Source: CAD feature listing. Evaluate the final solid. Frame: model axes, mm. A direction names the side the tool comes from. Give positions to 0.01 mm unless a question says otherwise; leave off trailing zeros. Order: outer loops, then holes, each group sorted by start corner. A loop starts at its lowest first (then second) coordinate and runs counter-clockwise, first axis right, second up. Notation, with made-up numbers: (48, 74) - (72, 74) arc R27 ccw to (72, 104) - close; hole circle Ø5 at (85, -8.75). An arc over 180 degrees is marked (long way). One line per item, written item: value. Start each with the question number.
Autodesk Inventor part; units mm, degrees
ref_plane "YZ Plane" through (0, 0, 0) normal (1, 0, 0) x (0, 1, 0)
ref_plane "XZ Plane" through (0, 0, 0) normal (0, 1, 0) x (-1, 0, 0)
ref_plane "XY Plane" through (0, 0, 0) normal (0, 0, 1) x (1, 0, 0)
sketch "Sketch1" plane through (0, 0, 0) normal (0, 0, 1) x (1, 0, 0)
  line L0 (0, 0) -> (0, -50.8)
  line L1 (0, -50.8) -> (-3.175, -50.8)
  line L2 (-3.175, -50.8) -> (-3.175, -3.175)
  line L3 (-3.175, -3.175) -> (-50.8, -3.175)
  line L4 (-50.8, -3.175) -> (-50.8, 0)
  line L5 (-50.8, 0) -> (0, 0)
  dimension "d0" = 50.8
  dimension "d1" = 3.175
  dimension "d2" = 47.625
  dimension "d3" = 47.625
extrude "Extrusion1" add sketch "Sketch1" along normal blind 50.8
sketch "Sketch2" plane through (-3.175, -50.8, 0) normal (-1, 0, 0) x (0, 0, 1)
  circle A0 centre (25.4, 22.225) radius 9.525
  line L0 (0, 50.8) -> (0, 0)
  line L1 (0, 0) -> (50.8, 0)
  circle A1 centre (25.4, 22.225) radius 25.4 construction
  circle A2 centre (44.8818, 38.5228) radius 2.3813
  circle A3 centre (5.9223, 5.9223) radius 2.3813
  line L2 (5.9223, 5.9223) -> (5.9223, 50.8) construction
  line L3 (0, 50.8) -> (50.8, 50.8) construction
  line L4 (5.9223, 5.9223) -> (0, 5.9223) construction
  line L5 (5.9223, 5.9223) -> (5.9223, 0) construction
  line L6 (50.8, 0) -> (50.8, 50.8) construction
  dimension "d9" = 25.4
  dimension "d10" = 22.225
  dimension "d13" = 50.8
  dimension "d14" = 4.7625
  dimension "d15" = 4.7625
  dimension "d16" = 5.9182
  dimension "d17" = 19.05
extrude "Extrusion2" cut sketch "Sketch2" against normal blind 3.175
properties part number "bag motor bracket"
1. Set-up query: faces 1 (the flat face through (-27, -3.175, 25)), 2 (the flat face through (-14, -3, 0)). Return all of +Z, -Z, +X, -X, +Y, -Y with unobstructed straight access to the full face (end or side cutting, diameter ignored); none if empty.
2. Section B-B on y = -29.5. Return the cut outline in (x, z) (3 decimals).
3. Draft query along Z for faces 3 (the flat face through (-2, -50.8, 25)), 4 (the flat face through (-14, -3, 50.8)), 5 (the cylindrical face through (-1.6, -12.2, 42.5)). Return one class per face: pulls with the +Z half, pulls with the -Z half, needs draft (parallel to the pull), parting line crosses it, or undercut.
4. Section A-A on z = 25.4. Return the cut outline in (x, y) (3 decimals).
5. Section D-D on y = -21.5. Return the cut outline in (x, z) (3 decimals).
6. Ray query, L1, parallel to Y at x = -2, z = 25; L2, parallel to Y at x = -23.5, z = 26 (3 decimals). Return the intervals inside material, ascending.
7. Section C-C on z = 37. Return the cut outline in (x, y) (3 decimals).
8. Contact query for flat-ended pins moving along their axis: pin 1 Ø5.5 at (y, z) = (-12.28, 44.88) entering from -X (3 decimals); pin 2 Ø6 at (x, z) = (-8, 21.5) entering from -Y (3 decimals). Output: stop coordinate, or through.
Data:
1. face 1: +Z, -Z, -X, -Y
1. face 2: -Z, +X, -X, +Y, -Y
2. outline: (-3.175, 0) - (0, 0) - (0, 15.92) - (-3.175, 15.92) - close; (-3.175, 34.88) - (0, 34.88) - (0, 50.8) - (-3.175, 50.8) - close
3. face 3: needs draft
3. face 4: pulls with the +Z half
3. face 5: undercut
4. outline: (-50.8, -3.175) - (-3.175, -3.175) - (-3.175, -19.05) - (0, -19.05) - (0, 0) - (-50.8, 0) - close; (-3.175, -50.8) - (0, -50.8) - (0, -38.1) - (-3.175, -38.1) - close
5. outline: (-3.175, 0) - (0, 0) - (0, 19.023) - (-3.175, 19.023) - close; (-3.175, 31.777) - (0, 31.777) - (0, 50.8) - (-3.175, 50.8) - close
6. L1: y = -50.8 to -38.09, -19.06 to 0
6. L2: y = -3.175 to 0
7. outline: (-50.8, -3.175) - (-3.175, -3.175) - (-3.175, -50.8) - (0, -50.8) - (0, 0) - (-50.8, 0) - close
8. pin 1: stops at x = -3.175
8. pin 2: stops at y = -3.175
